Here's how the part is built. I have some questions about the finished solid (model axes, mm). Face numbers are marked on the shaded views. A direction names the side the tool comes from. Coordinates: 2 decimals unless noted, no trailing zeros. Write each loop counter-clockwise with the first axis right and the second up, starting at its lowest first coordinate (ties: lowest second). Pieces come first, ordered by that corner, then holes.
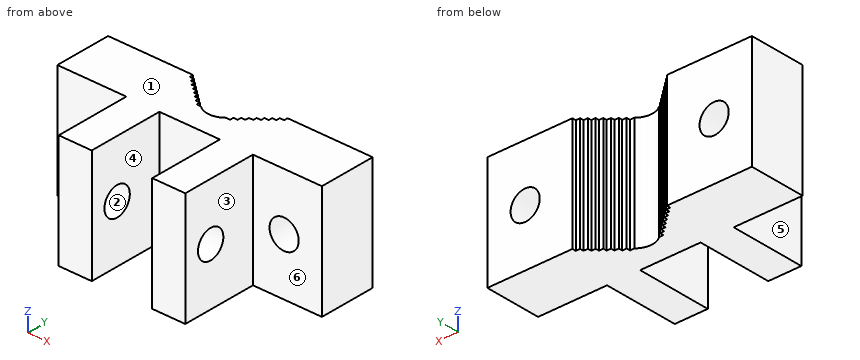
```python
from build123d import *

# Parameters (mm, degrees)
SKETCH1_W                    = 88.9
SKETCH1_H                    = 19.05
BOSS_EXTRUDE1_DEPTH          = 38.1
CUT_EXTRUDE1_REACH           = 40.1
F_3_8_CLEARANCE_HOLE1_D      = 9.8044
SKETCH7_W                    = 11.1125
SKETCH7_H                    = 38.1
BOSS_EXTRUDE2_DEPTH          = 25.4
F_3_8_0_375_DIAMETER_HOLE1_D = 9.525


with BuildPart() as part:
    # Sketch1 → Boss-Extrude1 (new body)
    with BuildSketch(Plane.XY):
        with Locations((0, 9.525)):
            Rectangle(SKETCH1_W, SKETCH1_H)
    extrude(amount=-BOSS_EXTRUDE1_DEPTH)

    # Sketch2 → Cut-Extrude1 (cut, up to next)
    with BuildSketch(Plane.XY, mode=Mode.PRIVATE) as cut_extrude1_sk1:
        with BuildLine():
            Line((-15.875, 19.05), (0, 19.05))
            Line((0, 19.05), (15.875, 19.05))
            Line((15.875, 19.05), (15.875, 17.78))
            Line((15.875, 17.78), (14.410694861, 17.78))
            Line((14.410694861, 17.78), (14.410694861, 16.51))
            Line((14.410694861, 16.51), (12.946389723, 16.51))
            Line((12.946389723, 16.51), (12.946389723, 15.24))
            Line((12.946389723, 15.24), (11.482084584, 15.24))
            Line((11.482084584, 15.24), (11.482084584, 13.97))
            Line((11.482084584, 13.97), (10.017779445, 13.97))
            Line((10.017779445, 13.97), (10.017779445, 12.7))
            Line((10.017779445, 12.7), (8.553474306, 12.7))
            Line((8.553474306, 12.7), (8.553474306, 11.43))
            Line((8.553474306, 11.43), (7.089169168, 11.43))
            Line((7.089169168, 11.43), (7.089169168, 10.16))
            Line((7.089169168, 10.16), (5.624864029, 10.16))
            Line((5.624864029, 10.16), (5.624864029, 8.89))
            Line((5.624864029, 8.89), (4.16055889, 8.89))
            ThreePointArc((4.16055889, 8.89), (0, 7.337108475), (-4.16055889, 8.89))
            Line((-4.16055889, 8.89), (-5.624864029, 8.89))
            Line((-5.624864029, 8.89), (-5.624864029, 10.16))
            Line((-5.624864029, 10.16), (-7.089169168, 10.16))
            Line((-7.089169168, 10.16), (-7.089169168, 11.43))
            Line((-7.089169168, 11.43), (-8.553474306, 11.43))
            Line((-8.553474306, 11.43), (-8.553474306, 12.7))
            Line((-8.553474306, 12.7), (-10.017779445, 12.7))
            Line((-10.017779445, 12.7), (-10.017779445, 13.97))
            Line((-10.017779445, 13.97), (-11.482084584, 13.97))
            Line((-11.482084584, 13.97), (-11.482084584, 15.24))
            Line((-11.482084584, 15.24), (-12.946389723, 15.24))
            Line((-12.946389723, 15.24), (-12.946389723, 16.51))
            Line((-12.946389723, 16.51), (-14.410694861, 16.51))
            Line((-14.410694861, 16.51), (-14.410694861, 17.78))
            Line((-14.410694861, 17.78), (-15.875, 17.78))
            Line((-15.875, 17.78), (-15.875, 19.05))
        make_face()
    cut_extrude1_tool1 = extrude(cut_extrude1_sk1.sketch, amount=-CUT_EXTRUDE1_REACH, mode=Mode.PRIVATE) & part.part
    add(cut_extrude1_tool1.solids().sort_by_distance((0, 14.620592, 0))[0], mode=Mode.SUBTRACT)

    # 3/8 Clearance Hole1 (through all)
    with Locations(Plane(origin=(0, 19.05, 0), x_dir=(1, 0, 0), z_dir=(0, 1, 0))):
        with Locations((-31.75, 19.05), (31.75, 19.05)):
            Hole(F_3_8_CLEARANCE_HOLE1_D / 2)

    # Sketch7 → Boss-Extrude2 (add)
    with BuildSketch(Plane.XZ):
        with Locations((-15.71625, -19.05)):
            Rectangle(SKETCH7_W, SKETCH7_H)
        with Locations((15.71625, -19.05)):
            Rectangle(SKETCH7_W, SKETCH7_H)
    extrude(amount=BOSS_EXTRUDE2_DEPTH)

    # 3/8 (0.375) Diameter Hole1 (through all)
    with Locations(Plane(origin=(21.2725, 0, 0), x_dir=(0, 0, -1), z_dir=(1, 0, 0))):
        with Locations((19.05, -15.875)):
            Hole(F_3_8_0_375_DIAMETER_HOLE1_D / 2)


solid = part.part
```
1) I need wall thicknesses on probe 1 along X at (y, z) = (11, -19.05); probe 2 along X at (y, z) = (-14.5, -6.5); probe 3 along Y at (x, z) = (14, -19.05). Which ranges of each line are inside material? Lowest first, please.
Values follow:
probe 1: x = -44.45 to -36.65, -26.85 to -7.09, 7.09 to 26.85, 36.65 to 44.45
probe 2: x = -21.27 to -10.16, 10.16 to 21.27
probe 3: y = -25.4 to -20.64, -11.11 to 16.51
2) Imagine slicing it at C-C on y = 2. Please give me the cut outline in (x, z).
Values follow:
outline: (-44.45, -38.1) - (44.45, -38.1) - (44.45, 0) - (-44.45, 0) - close; hole circle Ø9.8 at (-31.75, -19.05); hole circle Ø9.8 at (31.75, -19.05)
3) Imagine slicing it at B-B on y = -22. Please give me the cut outline in (x, z).
Values follow:
outline: (-21.27, -38.1) - (-10.16, -38.1) - (-10.16, 0) - (-21.27, 0) - close; (10.16, -38.1) - (21.27, -38.1) - (21.27, 0) - (10.16, 0) - close
4) We'd pull the mould along Z, two halves only. Please class the marked faces 1, 2 and 3: pulls with the +Z half, pulls with the -Z half, needs draft (parallel to the pull), parting line crosses it, or undercut.
Values follow:
face 1: pulls with the +Z half
face 2: undercut
face 3: needs draft
5) Imagine slicing it at D-D on z = -19.05. Count the separate pieces of the cut face and the enclosed holes in it, then the cut area to 3 significant figures.
Values follow:
separate pieces: 5
enclosed holes: 0
area: 1,450 mm2
6) Will these pins go through, and if not, where does the flat tip stop? pin 1 (3 mm diameter, centred on y = -11, z = -14, fed in from +X); pin 2 (1.6 mm diameter, centred on x = -12.5, z = -22.5, fed in from +Y); pin 3 (18.5 mm diameter, centred on x = 36.5, z = -23, fed in from -Y); pin 4 (10 mm diameter, centred on x = 3, y = -6, fed in from -Z).
Values follow:
pin 1: stops at x = 21.27
pin 2: stops at y = 16.51
pin 3: stops at y = 0
pin 4: passes through
7) Imagine slicing it at A-A on x = -31.75. Please give me the cut outline in (y, z), then the cut area to 3 significant figures.
Values follow:
outline: (0, -38.1) - (19.05, -38.1) - (19.05, -23.95) - (0, -23.95) - close; (0, -14.15) - (19.05, -14.15) - (19.05, 0) - (0, 0) - close
area: 539 mm2
8) On a 3-axis mill with a long thin cutter (end or side, diameter ignored), from which of +Z, -Z, +X, -X, +Y, -Y can I reach the whole of each face in a straight line? I mean the marked faces 4, 5 and 6. Say none if no direction works.
Values follow:
face 4: +Z, -Z, -Y
face 5: +Z, -Z, -X, -Y
face 6: +Z, -Z, +X, -Y
